Can you work these out from the drawing? Everything is in mm from the part's minimum corner. A direction names the side the tool comes from. Round coordinates to 2 decimals unless told otherwise and drop trailing zeros. Loops run counter-clockwise (first coordinate to the right, second up) from the corner with the lowest first, then second, coordinate; pieces in that order, holes last. Notation, with made-up numbers: M 56.25,50.25 L 69.25,50.25 A22 cw 69.25,81.25 Z; hole C 75.5,68.25 d4. An arc over 180 degrees is marked long. Use a Markdown table: item, result.
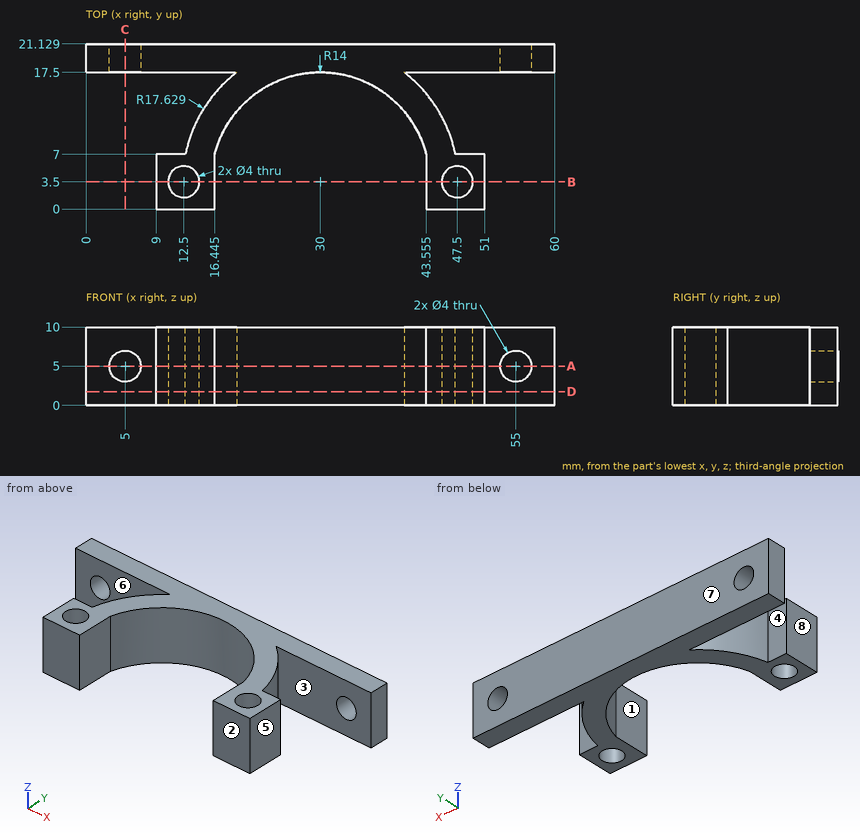
1. We'd pull the mould along Y, two halves only. Please class the marked faces 6, 7 and 8: +Y half, -Y half, draft (parallel to the pull), parting line (faces both ways), or undercut.
Answer sheet:
| item | result |
|---|---|
| face 6 | undercut |
| face 7 | +Y half |
| face 8 | draft |
2. Imagine slicing it at D-D, the plane z = 1.75. Write out the boundary of the cut face in (x, y) (1 decimal).
Answer sheet:
| item | result |
|---|---|
| outline | M 0,17.5 L 19.3,17.5 A17.6 ccw 12.7,7 L 9,7 L 9,0 L 16.4,0 L 16.4,7 A14 cw 43.6,7 L 43.6,0 L 51,0 L 51,7 L 47.3,7 A17.6 ccw 40.7,17.5 L 60,17.5 L 60,21.1 L 0,21.1 Z; hole C 12.5,3.5 d4; hole C 47.5,3.5 d4 |
3. Imagine slicing it at B-B, the plane y = 3.5. Write out the boundary of the cut face in (x, z) (1 decimal).
Answer sheet:
| item | result |
|---|---|
| outline | M 9,0 L 10.5,0 L 10.5,10 L 9,10 Z; M 14.5,0 L 16.4,0 L 16.4,10 L 14.5,10 Z; M 43.6,0 L 45.5,0 L 45.5,10 L 43.6,10 Z; M 49.5,0 L 51,0 L 51,10 L 49.5,10 Z |
4. Imagine slicing it at C-C, the plane x = 5. Write out the boundary of the cut face in (y, z).
Answer sheet:
| item | result |
|---|---|
| outline | M 17.5,0 L 21.13,0 L 21.13,3 L 17.5,3 Z; M 17.5,7 L 21.13,7 L 21.13,10 L 17.5,10 Z |
5. Which directions (+Z, -Z, +X, -X, +Y, -Y) give clear straight access to the entire face, cutting with the end or side of a thin tool? Please do the marked faces 1, 2, 3, 4 and 5.
Answer sheet:
| item | result |
|---|---|
| face 1 | +Z, -Z, -Y |
| face 2 | +Z, -Z, +X, -X, -Y |
| face 3 | +Z, -Z, +X |
| face 4 | +Z, -Z, -X |
| face 5 | +Z, -Z, +X, -Y |
6. I need wall thicknesses on probe 1 along Y at (x, z) = (12.5, 3.5); probe 2 along Y at (x, z) = (50.5, 0.75); probe 3 along X at (y, z) = (1.25, 1.5) (1 decimal). Which ranges of each line are inside material? Lowest first, please. Write a range as from..to.
Answer sheet:
| item | result |
|---|---|
| probe 1 | 0..1.5, 5.5..7, 17.5..21.13 |
| probe 2 | 0..7, 17.5..21.13 |
| probe 3 | 9..16.4, 43.6..51 |
7. Imagine slicing it at A-A, the plane z = 5. Write out the boundary of the cut face in (x, y) (1 decimal).
Answer sheet:
| item | result |
|---|---|
| outline | M 0,17.5 L 3,17.5 L 3,21.1 L 0,21.1 Z; M 7,17.5 L 19.3,17.5 A17.6 ccw 12.7,7 L 9,7 L 9,0 L 16.4,0 L 16.4,7 A14 cw 43.6,7 L 43.6,0 L 51,0 L 51,7 L 47.3,7 A17.6 ccw 40.7,17.5 L 53,17.5 L 53,21.1 L 7,21.1 Z; M 57,17.5 L 60,17.5 L 60,21.1 L 57,21.1 Z; hole C 12.5,3.5 d4; hole C 47.5,3.5 d4 |
8. For pin 1 Ø3 at (x, y) = (52, 17.5) entering from -Z; pin 2 Ø2 at (y, z) = (3.5, 7) entering from -X; pin 3 Ø1 at (y, z) = (16, 9) entering from +X (1 decimal); pin 4 Ø5.5 at (y, z) = (4, 6.5) entering from +X, each with a flat end and sliding along its axis, tell me the tip position at first contact or that it passes through.
Answer sheet:
| item | result |
|---|---|
| pin 1 | z = 0 |
| pin 2 | x = 9 |
| pin 3 | x = 42.9 |
| pin 4 | x = 51 |
